from build123d import *

# Parameters (mm, degrees)
F0_W     = 15
F0_H     = 15
F1_DEPTH = 7
F2_R     = 1.5
F3_DEPTH = 15
F4_R     = 1.5
F5_DEPTH = 15
F6_W     = 3
F6_H     = 3
F7_DEPTH = 3
F8_R     = 2.5
F9_DEPTH = 6
F10_R    = 2.5


with BuildPart() as f1:
    # F0 (on Front) → F1 (new body)
    with BuildSketch(Plane.XZ):
        with Locations((4.360599, 2.854392)):
            Rectangle(F0_W, F0_H)
    extrude(amount=F1_DEPTH)

    # F2 (on face) → F3 (cut)
    with BuildSketch(Plane.XY.offset(10.354392)):
        with Locations((-0.639401, -3.5)):
            Circle(F2_R)
    extrude(amount=-F3_DEPTH, mode=Mode.SUBTRACT)

    # F4 (on face) → F5 (cut)
    with BuildSketch(Plane.XY.offset(10.354392)):
        with Locations((9.360599, -3.5)):
            Circle(F4_R)
    extrude(amount=-F5_DEPTH, mode=Mode.SUBTRACT)

    # F6 (on face) → F7 (join)
    with BuildSketch(Plane.XZ.offset(7)):
        with Locations((4.070706, 3.2569)):
            Rectangle(F6_W, F6_H)
    extrude(amount=F7_DEPTH)

    # F8 (on face) → F9 (join)
    with BuildSketch(Plane(origin=(0, 0, 0), x_dir=(-1, 0, 0), z_dir=(0, 1, 0))):
        with Locations((-4.360599, 2.854392)):
            Circle(F8_R)
    extrude(amount=F9_DEPTH)

    # F10
    f10_edges = [f1.edges().sort_by_distance(p)[0] for p in [
        (6.860599, 6, 2.854392),
    ]]
    fillet(f10_edges, radius=F10_R)


solid = f1.part
Geometry: final body of the model. Coordinates: model frame, mm. A direction names the side the tool comes from. Give positions to 0.01 mm unless a question says otherwise; leave off trailing zeros. Order: outer loops, then holes, each group sorted by start corner. A loop starts at its lowest first (then second) coordinate and runs counter-clockwise, first axis right, second up. Notation, with made-up numbers: (79.25, 57.5) -> (89.25, 57.5) arc R27 cw to (89.25, 81.5) -> close; hole circle Ø4 at (11.25, 61). An arc over 180 degrees is marked (long way). Answer as a JSON object with one key per item and string values.
Q1. Section B-B (z = 6.75). Output: boundary loops of the cut face in (x, y), plus the area to 3 significant figures.
Entries:
{"outline": "(-3.14, -7) -> (11.86, -7) -> (11.86, 0) -> (-3.14, 0) -> close; hole circle Ø3 at (-0.64, -3.5); hole circle Ø3 at (9.36, -3.5)", "area": "90.9 mm^2"}
Q2. Section C-C (x = -1.75). Output: boundary loops of the cut face in (y, z), plus the area to 3 significant figures.
Entries:
{"outline": "(-7, -4.65) -> (-4.51, -4.65) -> (-4.51, 10.35) -> (-7, 10.35) -> close; (-2.49, -4.65) -> (0, -4.65) -> (0, 10.35) -> (-2.49, 10.35) -> close", "area": "74.8 mm^2"}
Q3. Section A-A (y = -3.5). Output: boundary loops of the cut face in (x, z).
Entries:
{"outline": "(-3.14, -4.65) -> (-2.14, -4.65) -> (-2.14, 10.35) -> (-3.14, 10.35) -> close; (0.86, -4.65) -> (7.86, -4.65) -> (7.86, 10.35) -> (0.86, 10.35) -> close; (10.86, -4.65) -> (11.86, -4.65) -> (11.86, 10.35) -> (10.86, 10.35) -> close"}
Q4. Access query for faces 4 (the flat face through (4, -8, 1.757)), 5 (the cylindrical face through (6.86, 1.73, 2.96)), 6 (the flat face through (2.571, -8, 3)), 7 (the flat face through (5.571, -8, 3)). Directions: +Z, -Z, +X, -X, +Y, -Y. A direction counts if a zero-diameter tool reaches every point of the face in a straight line with its end or side. Return the directions, or none.
Entries:
{"face 4": "-Z, +X, -X, -Y", "face 5": "+Y", "face 6": "+Z, -Z, -X, -Y", "face 7": "+Z, -Z, +X, -Y"}
Q5. Section D-D (z = 4). Output: boundary loops of the cut face in (x, y).
Entries:
{"outline": "(-3.14, -7) -> (2.57, -7) -> (2.57, -10) -> (5.57, -10) -> (5.57, -7) -> (11.86, -7) -> (11.86, 0) -> (6.58, 0) -> (6.58, 3.5) arc R2.22 ccw to (2.14, 3.5) -> (2.14, 0) -> (-3.14, 0) -> close; hole circle Ø3 at (-0.64, -3.5); hole circle Ø3 at (9.36, -3.5)"}
Q6. Material intervals for probe 1 along Y at (x, z) = (9.25, 1.5); probe 2 along X at (y, z) = (-4, 4.5); probe 3 along Y at (x, z) = (8, 3.5), sorted ascending.
Entries:
{"probe 1": "y = -7 to -5, -2 to 0", "probe 2": "x = -3.14 to -2.05, 0.77 to 7.95, 10.77 to 11.86", "probe 3": "y = -7 to -4.13, -2.87 to 0"}
Q7. First-contact query: pin 1 (2.5 mm diameter, centred on x = -0.64, y = -3.5, fed in from +Z); pin 2 (3.5 mm diameter, centred on y = -8, z = 3.5, fed in from +X); pin 3 (5 mm diameter, centred on x = 1, z = 2, fed in from +Y); pin 4 (1 mm diameter, centred on x = 6, z = -3, fed in from -Y). Flat tips, straight axial feed; report the tip coordinate or a pass-through.
Entries:
{"pin 1": "passes through", "pin 2": "stops at x = 11.86", "pin 3": "stops at y = 5.81", "pin 4": "stops at y = -7"}
Q8. Draft query along Y for faces 1 (the flat face through (4, -8, 4.757)), 2 (the cylindrical face through (8.255, -2.486, 2.959)), 3 (the flat face through (1, 0, 3)). Return one class per face: released by +Y, released by -Y, zero draft, split by the parting line, or undercut.
Entries:
{"face 1": "zero draft", "face 2": "undercut", "face 3": "released by +Y"}
